Design review of the part built by this model. Coordinates are the model's own, in mm. A direction names the side the tool comes from. Give positions to 0.01 mm unless a question says otherwise; leave off trailing zeros. Loops run counter-clockwise (first coordinate to the right, second up) from the corner with the lowest first, then second, coordinate; pieces in that order, holes last. Notation, with made-up numbers: (-9, 2) - (3, 2) arc R16 cw to (3, 8) - close; hole circle Ø7 at (36, -21.5). An arc over 180 degrees is marked (long way). Write each question's results on one line, items separated by ' | '.
from build123d import *

# Parameters (mm, degrees)
SKETCH_1_W      = 3.5
SKETCH_1_H      = 3
SKETCH_1_W_2    = 3
SKETCH_1_H_2    = 3.5
EXTRUDE_1_DEPTH = 3
FILLET_1_R      = 1.5


with BuildPart() as part:
    # Эскиз1 → Бобышка-Вытянуть1 (new body)
    with BuildSketch(Plane.XY):
        Polygon((0, 22.492640687), (0, 0), (-22.492640687, 0), align=None)
        with Locations((-11.5, 3.5)):
            Rectangle(SKETCH_1_W, SKETCH_1_H, mode=Mode.SUBTRACT)
        with Locations((-3.5, 11.5)):
            Rectangle(SKETCH_1_W_2, SKETCH_1_H_2, mode=Mode.SUBTRACT)
    extrude(amount=EXTRUDE_1_DEPTH)

    # Скругление1
    fillet_1_edges = [part.edges().sort_by_distance(p)[0] for p in [
        (0, 0, 1.5),
        (-22.492640687, 0, 1.5),
        (0, 22.492640687, 1.5),
    ]]
    fillet(fillet_1_edges, radius=FILLET_1_R)


solid = part.part
(1) Take a section at B-B on x = -3.75. Give the boundary of the cut face in (y, z), plus the area to 3 significant figures.
Answers below:
outline: (0, 0) - (9.75, 0) - (9.75, 3) - (0, 3) - close; (13.25, 0) - (18.74, 0) - (18.74, 3) - (13.25, 3) - close | area: 45.7 mm2
(2) Wall thickness on line 1 along Y through (x, z) = (-2.25, 1.45); line 2 along Y through (x, z) = (-4.25, 2.4); line 3 along X through (y, z) = (4.75, 2.15): over which ranges is each line inside the solid? List them lowest first. Write a range as from..to.
Answers below:
line 1: 0..9.75, 13.25..20.17 | line 2: 0..9.75, 13.25..18.24 | line 3: -17.74..-13.25, -9.75..0
(3) Tool access review of faces 4 (the flat face through (-12, 5, 1)), 5 (the flat face through (-10, 0, 1)): name each direction out of +Z, -Z, +X, -X, +Y, -Y from which nothing blocks a thin tool from reaching the whole face with its end or side.
Answers below:
face 4: +Z, -Z | face 5: +Z, -Z, +X, -X, -Y
(4) Draft analysis for pull direction Y (two halves, no side actions). For faces 1 (the cylindrical face through (-0.43, 0.45, 1.52)), 2 (the flat face through (-11.37, 11.12, 1.48)), 3 (the flat face through (-9.75, 3, 1)), state which applies: pulls with the +Y half, pulls with the -Y half, needs draft (parallel to the pull), parting line crosses it, or undercut.
Answers below:
face 1: pulls with the -Y half | face 2: pulls with the +Y half | face 3: undercut
(5) Take a section at D-D on x = -11. Give the boundary of the cut face in (y, z), plus the area to 3 significant figures.
Answers below:
outline: (0, 0) - (2, 0) - (2, 3) - (0, 3) - close; (5, 0) - (11.49, 0) - (11.49, 3) - (5, 3) - close | area: 25.5 mm2
(6) Take a section at C-C on y = 16.25. Give the boundary of the cut face in (x, z), plus the area to 3 significant figures.
Answers below:
outline: (-6.24, 0) - (0, 0) - (0, 3) - (-6.24, 3) - close | area: 18.7 mm2
(7) Take a section at A-A on z = 1.8. Give the boundary of the cut face in (x, y).
Answers below:
outline: (-19.93, 2.56) arc R1.5 ccw to (-18.87, 0) - (-1.5, 0) arc R1.5 ccw to (0, 1.5) - (0, 18.87) arc R1.5 ccw to (-2.56, 19.93) - close; hole (-13.25, 2) - (-9.75, 2) - (-9.75, 5) - (-13.25, 5) - close; hole (-5, 9.75) - (-2, 9.75) - (-2, 13.25) - (-5, 13.25) - close
(8) Insertion check: P1, Ø1.5, axis at x = -16, y = 8, coming from the -Z side; P2, Ø0.9, axis at x = -11, z = 2, coming from the +Y side. Each pin has a flat end and moves straight along its axis. Give the tip position at first contact, or say it passes through.
Answers below:
P1: through | P2: y = 11.94
